```python
from build123d import *

# Parameters (mm, degrees)
SKETCH_2_W          = 170
SKETCH_2_H          = 20
EXTRUDE_1_DEPTH     = 23
CUT_EXTRUDE_1_DEPTH = 173.710740836
SKETCH_4_W          = 17
SKETCH_4_H          = 13
CUT_EXTRUDE_2_DEPTH = 30
CUT_EXTRUDE_3_DEPTH = 173.710740836
SKETCH_6_W          = 67.5
SKETCH_6_H          = 3
SKETCH_6_W_2        = 15
SKETCH_6_H_2        = 14.5
CUT_EXTRUDE_4_DEPTH = 173.710740836
SKETCH_7_W          = 25.348417758
SKETCH_7_H          = 9.515527538
CUT_EXTRUDE_5_DEPTH = 33.295510524
SKETCH_8_W          = 27
SKETCH_8_H          = 5
SKETCH_8_R          = 1.25
EXTRUDE_2_DEPTH     = 3
CUT_EXTRUDE_START   = -3
SKETCH_8_3_R        = 2
CUT_EXTRUDE_6_DEPTH = 1.5


with BuildPart() as part:
    # 草图2 → 凸台-拉伸1 (new body)
    with BuildSketch(Plane(origin=(0, 0, 0), x_dir=(1, 0, 0), z_dir=(0, 1, 0))):
        with Locations((85, -10)):
            Rectangle(SKETCH_2_W, SKETCH_2_H)
    extrude(amount=EXTRUDE_1_DEPTH)

    # 草图3 → 切除-拉伸1 (cut, through all)
    with BuildSketch(Plane(origin=(0, 23, 0), x_dir=(1, 0, 0), z_dir=(0, 1, 0))):
        with BuildLine():
            ThreePointArc((161.6, -10), (159.341699476, -8.541699476), (158.941699476, -11.2))
            Line((158.941699476, -11.2), (161.058300524, -11.2))
            ThreePointArc((161.058300524, -11.2), (161.458300524, -10.658300524), (161.6, -10))
        make_face()
        with BuildLine():
            ThreePointArc((126.6, -10), (124.341699476, -8.541699476), (123.941699476, -11.2))
            Line((123.941699476, -11.2), (126.058300524, -11.2))
            ThreePointArc((126.058300524, -11.2), (126.458300524, -10.658300524), (126.6, -10))
        make_face()
    extrude(amount=-CUT_EXTRUDE_1_DEPTH, mode=Mode.SUBTRACT)

    # 草图4 → 切除-拉伸2 (cut)
    with BuildSketch(Plane(origin=(170, 0, 0), x_dir=(0, 0, -1), z_dir=(1, 0, 0))):
        with Locations((-8.5, 11.5)):
            Rectangle(SKETCH_4_W, SKETCH_4_H)
    extrude(amount=-CUT_EXTRUDE_2_DEPTH, mode=Mode.SUBTRACT)

    # 草图5 → 切除-拉伸3 (cut, through all)
    with BuildSketch(Plane(origin=(0, 23, 0), x_dir=(1, 0, 0), z_dir=(0, 1, 0))):
        with BuildLine():
            Line((117.5, -17), (117.5, -10))
            ThreePointArc((117.5, -10), (125, -2.5), (132.5, -10))
            Line((132.5, -10), (132.5, -17))
            Line((132.5, -17), (152.5, -17))
            Line((152.5, -17), (152.5, -10))
            ThreePointArc((152.5, -10), (160, -2.5), (167.5, -10))
            Line((167.5, -10), (167.5, -17))
            Line((167.5, -17), (170, -17))
            Line((170, -17), (170, 0))
            Line((170, 0), (0, 0))
            Line((0, 0), (0, -20))
            Line((0, -20), (102.5, -20))
            Line((102.5, -20), (102.5, -17))
            Line((102.5, -17), (117.5, -17))
        make_face()
    extrude(amount=-CUT_EXTRUDE_3_DEPTH, mode=Mode.SUBTRACT)

    # 草图6 → 切除-拉伸4 (cut, through all)
    with BuildSketch(Plane(origin=(0, 23, 0), x_dir=(1, 0, 0), z_dir=(0, 1, 0))):
        with Locations((136.25, -18.5)):
            Rectangle(SKETCH_6_W, SKETCH_6_H)
        with Locations((125, -9.75)):
            Rectangle(SKETCH_6_W_2, SKETCH_6_H_2)
    extrude(amount=-CUT_EXTRUDE_4_DEPTH, mode=Mode.SUBTRACT)


with BuildPart() as cut_extrude_4_piece_1:
    # of the separate pieces the step leaves, piece 1, a body of its own (cut_extrude_4_pieces)
    add(part.part.solids().sort_by_distance((167.5, 23, 10))[0])

    # 草图7 → 切除-拉伸5 (cut, through all)
    with BuildSketch(Plane.ZY.offset(-152.5)):
        with Locations((10.223802201, 19.727293576)):
            Rectangle(SKETCH_7_W, SKETCH_7_H)
    extrude(amount=-CUT_EXTRUDE_5_DEPTH, mode=Mode.SUBTRACT)


with BuildPart() as cut_extrude_4_piece_2:
    # of the separate pieces the step leaves, piece 2, a body of its own (cut_extrude_4_pieces)
    add(part.part.solids().sort_by_distance((167.5, 0, 17))[0])

    # 草图8 → 凸台-拉伸2 (add)
    with BuildSketch(Plane.XY.offset(17)):
        with Locations((160, 2.5)):
            Rectangle(SKETCH_8_W, SKETCH_8_H)
        with Locations((149.5, 2.5)):
            Circle(SKETCH_8_R, mode=Mode.SUBTRACT)
        with Locations((170.5, 2.5)):
            Circle(SKETCH_8_R, mode=Mode.SUBTRACT)
    extrude(amount=-EXTRUDE_2_DEPTH)

    # 草图8<3> → 切除-拉伸6 (cut)
    with BuildSketch(Plane.XY.offset(17).offset(CUT_EXTRUDE_START)):
        with Locations((170.5, 2.5)):
            Circle(SKETCH_8_3_R)
        with Locations((149.5, 2.5)):
            Circle(SKETCH_8_3_R)
    extrude(amount=CUT_EXTRUDE_6_DEPTH, mode=Mode.SUBTRACT)


solid = cut_extrude_4_piece_2.part
```
Build history of the part. All positions in model axes, mm. A direction names the side the tool comes from. Round coordinates to 2 decimals unless told otherwise and drop trailing zeros. Write each loop counter-clockwise with the first axis right and the second up, starting at its lowest first coordinate (ties: lowest second). Pieces come first, ordered by that corner, then holes. Notation, with made-up numbers: (7, -19) - (18, -19) arc R32 ccw to (18, 15) - close; hole circle Ø9 at (26.5, 38). An arc over 180 degrees is marked (long way). Write each question's results on one line, items separated by ' | '. Start each with the question number.
Item 1: Saw through at A-A (y = 2.5). Write the cut outline in (x, z).
Item 2: Saw through at C-C (z = 16.25). Write the cut outline in (x, y), and give its area (3 significant figures).
Item 3: Which spindle directions (+Z, -Z, +X, -X, +Y, -Y) get a long thin tool onto all of the face, cutting with end or side? Do faces 1 (the face through (168.502, 2.588, 14.74)), 2 (the face through (160, 3, 11.2)), 3 (the face through (152.5, 3, 12)). Say none if no direction does.
Item 4: Saw through at B-B (x = 160). Write the cut outline in (y, z), and give its area (3 significant figures).
Item 5: Mould opens along X. For faces 4 (the face through (167.5, 3, 12)), 5 (the face through (168, 3, 14)), 6 (the face through (172, 3, 15.5)) say: pulls with the +X half, pulls with the -X half, needs draft (parallel to the pull), parting line crosses it, or undercut.
Item 6: Drop flat-ended pins along their axis: P1, Ø3, axis at y = 2.5, z = 12, coming from the +X side; P2, Ø1.5, axis at x = 149, y = 1.5, coming from the -Z side; P3, Ø1.2, axis at y = 2.5, z = 12, coming from the -X side. Give the stop position or say it passes through.
Item 7: Saw through at D-D (x = 170.5). Write the cut outline in (y, z).
Item 8: Wall check: L1, parallel to X at y = 3.6, z = 10; L2, parallel to Y at x = 170.5, z = 16.45; L3, parallel to Z at x = 147.5, y = 4. Give the ranges that are in metal, low to high. Write a range as [from, to].
Results are:
1) outline: (146.5, 14) - (147.5, 14) - (147.5, 15.5) - (148.25, 15.5) - (148.25, 17) - (146.5, 17) - close; (150.75, 15.5) - (151.5, 15.5) - (151.5, 14) - (152.5, 14) - (152.5, 10) arc R7.5 ccw to (167.5, 10) - (167.5, 14) - (168.5, 14) - (168.5, 15.5) - (169.25, 15.5) - (169.25, 17) - (150.75, 17) - close; (171.75, 15.5) - (172.5, 15.5) - (172.5, 14) - (173.5, 14) - (173.5, 17) - (171.75, 17) - close; hole (158.94, 11.2) arc R1.6 ccw (long way) to (161.06, 11.2) - close
2) outline: (146.5, 0) - (173.5, 0) - (173.5, 5) - (146.5, 5) - close; hole circle Ø2.5 at (149.5, 2.5); hole circle Ø2.5 at (170.5, 2.5) | area: 125 mm²
3) face 1: -Z | face 2: +Y, -Y | face 3: -Z, -X, +Y, -Y
4) outline: (0, 2.5) - (5, 2.5) - (5, 8.4) - (0, 8.4) - close; (0, 11.2) - (5, 11.2) - (5, 17) - (0, 17) - close | area: 58.5 mm²
5) face 4: pulls with the +X half | face 5: needs draft | face 6: undercut
6) P1: stops at x = 167.5 | P2: stops at z = 15.5 | P3: stops at x = 152.5
7) outline: (0, 14) - (0.5, 14) - (0.5, 15.5) - (1.25, 15.5) - (1.25, 17) - (0, 17) - close; (3.75, 15.5) - (4.5, 15.5) - (4.5, 14) - (5, 14) - (5, 17) - (3.75, 17) - close
8) L1: x = [152.5, 158.4], [161.6, 167.5] | L2: y = [0, 1.25], [3.75, 5] | L3: z = [14, 17]
